from build123d import *

# Parameters (mm, degrees)
PAD_DEPTH = 5


with BuildPart() as part:
    # Sketch → Pad (new body)
    with BuildSketch(Plane.XY):
        with BuildLine():
            ThreePointArc((-2, 9.287088), (0, -9.5), (2, 9.287088))
            Line((2, 9.287088), (2, 11.787088))
            ThreePointArc((2, 11.787088), (1.414214, 13.201301), (0, 13.787088))
            ThreePointArc((0, 13.787088), (-1.414214, 13.201301), (-2, 11.787088))
            Line((-2, 9.287088), (-2, 11.787088))
        make_face()
    extrude(amount=PAD_DEPTH)


solid = part.part
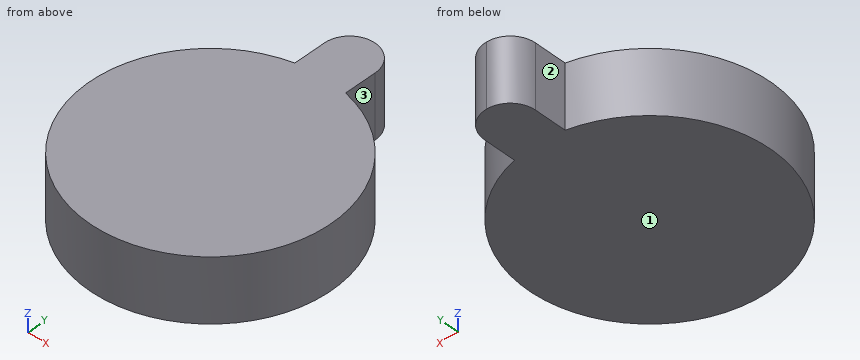
Could you check a few things on this model? Use its own coordinates, in mm. Face numbers are marked on the shaded views. A direction names the side the tool comes from. Coordinates: 2 decimals unless noted, no trailing zeros. Write each loop counter-clockwise with the first axis right and the second up, starting at its lowest first coordinate (ties: lowest second). Pieces come first, ordered by that corner, then holes. Notation, with made-up numbers: M 77,-25.5 L 116,-25.5 A32 cw 116,0.5 Z; hole C 29,-6.75 d1. An arc over 180 degrees is marked long. One line per question, with ' | ' between items.
1) For pin 1 Ø0.8 at (y, z) = (10, 3.5) entering from -X; pin 2 Ø2 at (y, z) = (-4.5, 4) entering from +X; pin 3 Ø3 at (x, z) = (-6, 2.5) entering from +Y, each with a flat end and sliding along its axis, tell me the tip position at first contact or that it passes through.
Checks:
pin 1: x = -2 | pin 2: x = 8.83 | pin 3: y = 8.37
2) Imagine slicing it at C-C, the plane y = 4. Write out the boundary of the cut face in (x, z).
Checks:
outline: M -8.62,0 L 8.62,0 L 8.62,5 L -8.62,5 Z
3) For the marked faces 1, 2 and 3, which set-ups out of +Z, -Z, +X, -X, +Y, -Y let a thin tool reach every point of the face, with its end or its side?
Checks:
face 1: -Z, +X, -X, +Y, -Y | face 2: +Z, -Z, -X, +Y | face 3: +Z, -Z, +X, +Y
4) I need wall thicknesses on probe 1 along X at (y, z) = (10.75, 0.5); probe 2 along Y at (x, z) = (-5, 2.9); probe 3 along Y at (x, z) = (0.75, 3.7). Which ranges of each line are inside material? Lowest first, please. Write a range as [from, to].
Checks:
probe 1: [-2, 2] | probe 2: [-8.08, 8.08] | probe 3: [-9.47, 13.64]
5) Imagine slicing it at B-B, the plane x = 1.25. Write out the boundary of the cut face in (y, z), and give its area (3 significant figures).
Checks:
outline: M -9.42,0 L 13.35,0 L 13.35,5 L -9.42,5 Z | area: 114 mm²
6) Imagine slicing it at A-A, the plane z = 1.8. Write out the boundary of the cut face in (x, y), and give its area (3 significant figures).
Checks:
outline: M -2,9.29 A9.5 ccw long 2,9.29 L 2,11.79 A2 ccw -2,11.79 Z | area: 299 mm²
